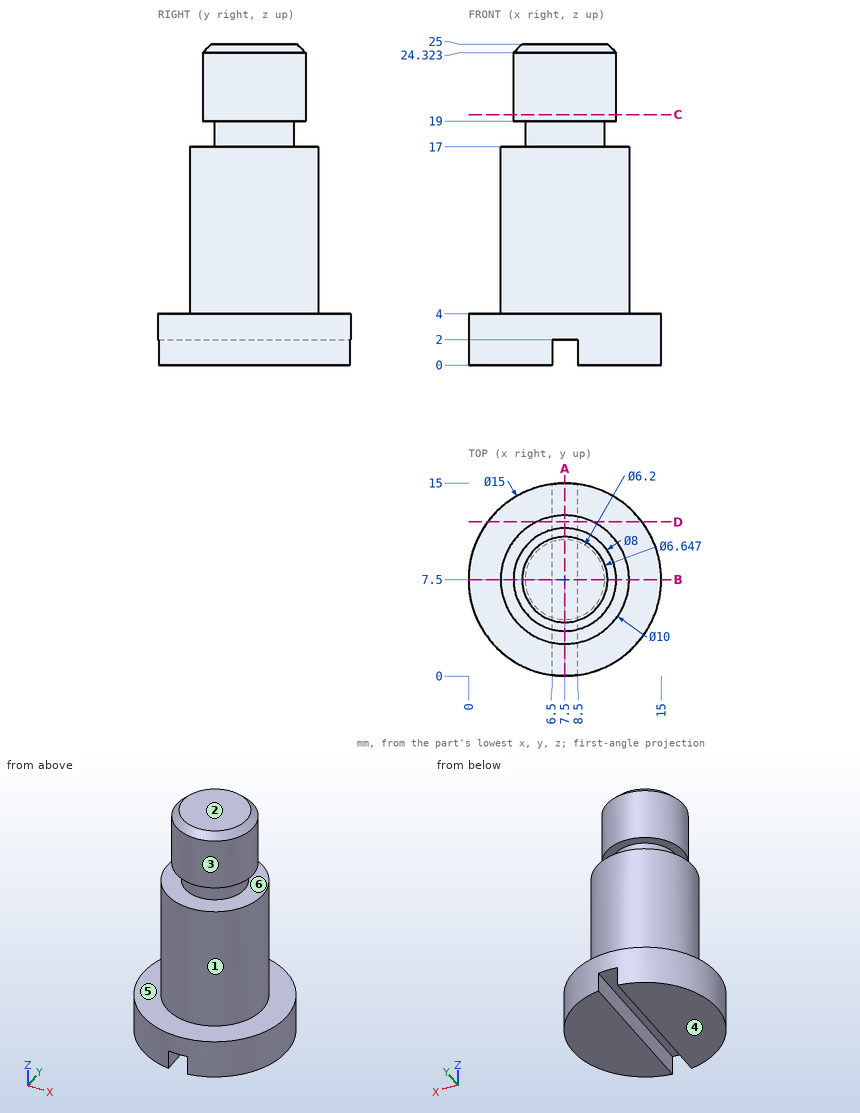
Job drawing, mm, ordinate dimensions from the low corner. One solid piece. A direction names the side the tool comes from. Give positions to 0.01 mm unless a question says otherwise; leave off trailing zeros. Loops run counter-clockwise (first coordinate to the right, second up) from the corner with the lowest first, then second, coordinate; pieces in that order, holes last.
Item 1: Drill centre lines: line 1 (Z direction, x = 4.5, y = 4.75); line 2 (Z direction, x = 14, y = 5); line 3 (Y direction, x = 6.25, z = 18.25) (1 decimal). Where is each one in solid material? Low to high.
Answers follow:
line 1: z = 0 to 17
line 2: z = 0 to 4
line 3: y = 4.7 to 10.3
Item 2: Slice it at D-D, the plane y = 12. List the corners of the cut face in (x, z).
Answers follow:
outline: (1.5, 0) - (6.5, 0) - (6.5, 2) - (8.5, 2) - (8.5, 0) - (13.5, 0) - (13.5, 4) - (9.68, 4) - (9.68, 17) - (5.32, 17) - (5.32, 4) - (1.5, 4) - close
Item 3: Slice it at A-A, the plane x = 7.5. List the corners of the cut face in (y, z), and give its area (3 significant figures).
Answers follow:
outline: (0, 2) - (15, 2) - (15, 4) - (12.5, 4) - (12.5, 17) - (10.6, 17) - (10.6, 19) - (11.5, 19) - (11.5, 24.32) - (10.82, 25) - (4.18, 25) - (3.5, 24.32) - (3.5, 19) - (4.4, 19) - (4.4, 17) - (2.5, 17) - (2.5, 4) - (0, 4) - close
area: 220 mm2
Item 4: Pull direction Z, two halves, no side cores. Call the marked faces 3, 4, 5 and 6: released by +Z, released by -Z, zero draft, split by the parting line, or undercut.
Answers follow:
face 3: zero draft
face 4: released by -Z
face 5: released by +Z
face 6: undercut
Item 5: Slice it at C-C, the plane z = 19.5. List the corners of the cut face in (x, y).
Answers follow:
outline: circle Ø8 at (7.5, 7.5)
Item 6: Flat gauge pins, fed straight in: pin 1 (6 mm diameter, centred on x = 7.5, z = 16.5, fed in from -Y); pin 2 (2 mm diameter, centred on y = 9.5, z = 1, fed in from +X); pin 3 (4 mm diameter, centred on y = 8, z = 17, fed in from -X). Where does each tip first touch, or does it go through?
Answers follow:
pin 1: stops at y = 2.5
pin 2: stops at x = 14.93
pin 3: stops at x = 2.5
Item 7: Slice it at B-B, the plane y = 7.5. List the corners of the cut face in (x, z).
Answers follow:
outline: (0, 0) - (6.5, 0) - (6.5, 2) - (8.5, 2) - (8.5, 0) - (15, 0) - (15, 4) - (12.5, 4) - (12.5, 17) - (10.6, 17) - (10.6, 19) - (11.5, 19) - (11.5, 24.32) - (10.82, 25) - (4.18, 25) - (3.5, 24.32) - (3.5, 19) - (4.4, 19) - (4.4, 17) - (2.5, 17) - (2.5, 4) - (0, 4) - close
Item 8: Which spindle directions (+Z, -Z, +X, -X, +Y, -Y) get a long thin tool onto all of the face, cutting with end or side? Do the marked faces 1 and 2. Say none if no direction does.
Answers follow:
face 1: +Z
face 2: +Z, +X, -X, +Y, -Y
